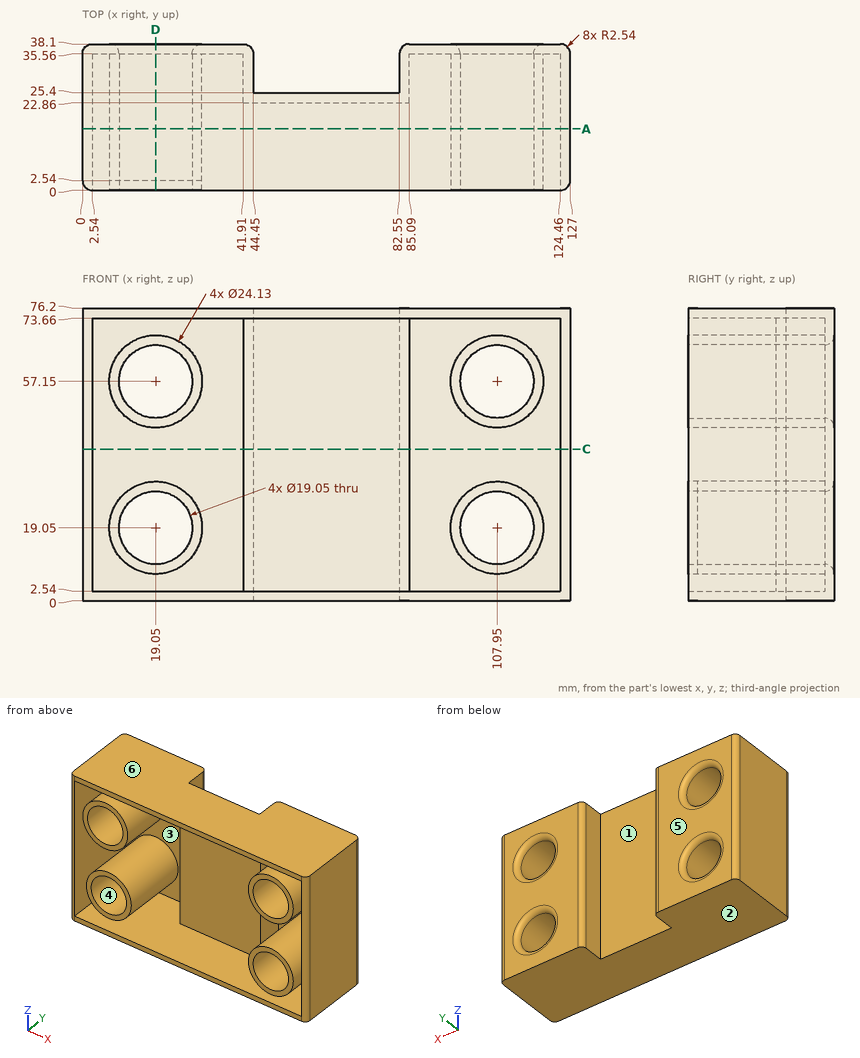
Could you check a few things on this drawing? It's one solid part, dimensions in mm from its lowest x, y, z. A direction names the side the tool comes from. Coordinates: 2 decimals unless noted, no trailing zeros. Loops run counter-clockwise (first coordinate to the right, second up) from the corner with the lowest first, then second, coordinate; pieces in that order, holes last. Notation, with made-up numbers: (26.5, 85) - (33.5, 85) arc R18 cw to (33.5, 93) - close; hole circle Ø11 at (71.5, 34). An arc over 180 degrees is marked (long way). Answer as a JSON object with one key per item and string values. Group by question number.
Item 1: If we section it at D-D (x = 19.05): List the corners of the cut face in (y, z) for me (3 decimals), plus the area to 3 significant figures.
Item 2: On a 3-axis mill with a long thin cutter (end or side, diameter ignored), from which of +Z, -Z, +X, -X, +Y, -Y can I reach the whole of each face in a straight line? I mean the marked faces 1, 2 and 3. Say none if no direction works.
Item 3: If I drill on L1, parallel to Z at x = 107.95, y = 12.5 (3 decimals); L2, parallel to X at y = 17, z = 19; L3, parallel to X at y = 36.5, z = 13.5, over which ranges is the centre line in solid material (lowest first)? Write a range as from..to.
Item 4: If we section it at A-A (y = 16): State how many separate pieces and enclosed holes the cut face has, plus the area to 3 significant figures.
Item 5: If we mould it in two halves opening along Z, with no side actions, what happens to the marked faces 4, 5 and 6? For each: released by +Z, released by -Z, zero draft, split by the parting line, or undercut.
Item 6: If we section it at C-C (z = 39.5): List the corners of the cut face in (x, y) for me, plus the area to 3 significant figures.
Returned:
{
 "1": {"outline": "(0, 0) - (38.1, 0) - (38.1, 6.985) arc R2.54 ccw to (35.56, 9.525) - (2.54, 9.525) - (2.54, 6.985) - (35.56, 6.985) - (35.56, 2.54) - (0, 2.54) - close; (0, 45.085) - (35.56, 45.085) - (35.56, 31.115) - (2.54, 31.115) - (2.54, 28.575) - (35.56, 28.575) arc R2.54 ccw to (38.1, 31.115) - (38.1, 45.085) arc R2.54 ccw to (35.56, 47.625) - (0, 47.625) - close; (0, 66.675) - (35.56, 66.675) arc R2.54 ccw to (38.1, 69.215) - (38.1, 76.2) - (0, 76.2) - (0, 73.66) - (35.56, 73.66) - (35.56, 69.215) - (0, 69.215) - close", "area": "620 mm²"},
 "2": {"face 1": "+Z, -Z, +Y", "face 2": "-Z, +X, -X, +Y, -Y", "face 3": "-Y"},
 "3": {"L1": "z = 0..2.54, 6.985..9.525, 28.575..31.115, 45.085..47.625, 66.675..69.215, 73.66..76.2", "L2": "x = 0..2.54, 6.99..9.53, 28.57..31.11, 95.89..98.43, 117.47..120.01, 124.46..127", "L3": "x = 0.18..11.09, 27.01..44.27, 82.73..99.99, 115.91..126.82"},
 "4": {"separate pieces": "5", "enclosed holes": "5", "area": "1,700 mm²"},
 "5": {"face 4": "undercut", "face 5": "zero draft", "face 6": "released by +Z"},
 "6": {"outline": "(0, 2.54) arc R2.54 ccw to (2.54, 0) - (2.54, 35.56) - (41.91, 35.56) - (41.91, 22.86) - (85.09, 22.86) - (85.09, 35.56) - (124.46, 35.56) - (124.46, 0) arc R2.54 ccw to (127, 2.54) - (127, 35.56) arc R2.54 ccw to (124.46, 38.1) - (85.09, 38.1) arc R2.54 ccw to (82.55, 35.56) - (82.55, 25.4) - (44.45, 25.4) - (44.45, 35.56) arc R2.54 ccw to (41.91, 38.1) - (2.54, 38.1) arc R2.54 ccw to (0, 35.56) - close", "area": "559 mm²"}
}
